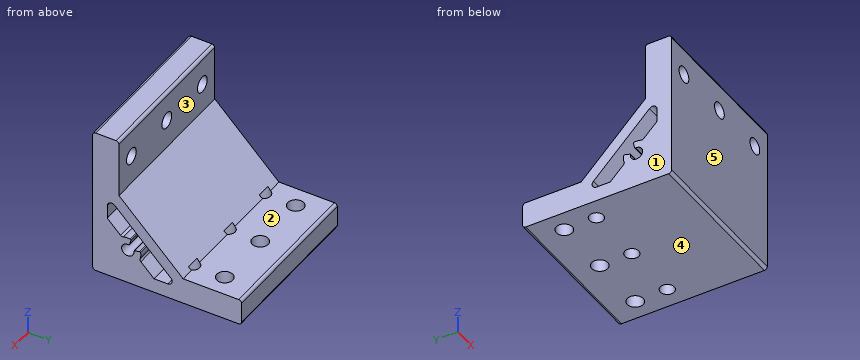
from build123d import *

# Parameters (mm, degrees)
BOSS_EXTRUDE1_DEPTH      = 27
BOSS_EXTRUDE1_DEPTH_BACK = 27
SKETCH6_R                = 2.75
CUT_EXTRUDE5_DEPTH       = 10
SKETCH7_R                = 2.75
CUT_EXTRUDE6_DEPTH       = 10
SKETCH9_R                = 2.4
CUT_EXTRUDE7_DEPTH       = 10


with BuildPart() as part:
    # Sketch1 → Boss-Extrude1 (new body, two sides)
    with BuildSketch(Plane(origin=(0, 0, 0), x_dir=(0, 0, -1), z_dir=(1, 0, 0))) as boss_extrude1_sk:
        with BuildLine():
            Line((-50, 0), (-1, 0))
            ThreePointArc((-1, 0), (-0.292893219, 0.292893219), (0, 1))
            Line((0, 1), (0, 50))
            ThreePointArc((0, 50), (-0.292893219, 50.707106781), (-1, 51))
            Line((-1, 51), (-8, 51))
            ThreePointArc((-8, 51), (-8.707106781, 50.707106781), (-9, 50))
            Line((-9, 50), (-9, 31))
            Line((-9, 31), (-31, 9))
            Line((-31, 9), (-50, 9))
            ThreePointArc((-50, 9), (-50.707106781, 8.707106781), (-51, 8))
            Line((-51, 8), (-51, 1))
            ThreePointArc((-51, 1), (-50.707106781, 0.292893219), (-50, 0))
        make_face()
        with BuildLine():
            Line((-25.721825407, 5), (-20.999285733, 5))
            Line((-20.999285733, 5), (-16.494036438, 9.505249294))
            ThreePointArc((-16.494036438, 9.505249294), (-16.226979866, 9.987090789), (-16.255625497, 10.537245192))
            ThreePointArc((-16.255625497, 10.537245192), (-16.488859314, 11.683547702), (-16.418755424, 12.851234691))
            ThreePointArc((-16.418755424, 12.851234691), (-16.283360667, 13.048766752), (-16.046526031, 13.084263382))
            Line((-16.046526031, 13.084263382), (-14.300039569, 12.616293745))
            ThreePointArc((-14.300039569, 12.616293745), (-14.127781033, 12.492491496), (-14.080474622, 12.285701498))
            ThreePointArc((-14.080474622, 12.285701498), (-10.515075745, 10.515075774), (-12.285701539, 14.080474617))
            ThreePointArc((-12.285701539, 14.080474617), (-12.492491514, 14.127781045), (-12.616293745, 14.300039569))
            Line((-12.616293745, 14.300039569), (-13.084263382, 16.046526031))
            ThreePointArc((-13.084263382, 16.046526031), (-13.048766728, 16.283360705), (-12.851234602, 16.418755442))
            ThreePointArc((-12.851234602, 16.418755442), (-11.683774102, 16.488875269), (-10.537674556, 16.255773055))
            ThreePointArc((-10.537674556, 16.255773055), (-9.987311976, 16.226928716), (-9.505249294, 16.494036438))
            Line((-9.505249294, 16.494036438), (-5, 20.999285733))
            Line((-5, 20.999285733), (-5, 25.721825407))
            ThreePointArc((-5, 25.721825407), (-5.925974851, 27.107644706), (-7.560660172, 26.782485579))
            Line((-7.560660172, 26.782485579), (-26.782485579, 7.560660172))
            ThreePointArc((-26.782485579, 7.560660172), (-27.107644706, 5.925974851), (-25.721825407, 5))
        make_face(mode=Mode.SUBTRACT)
    extrude(amount=BOSS_EXTRUDE1_DEPTH)
    extrude(boss_extrude1_sk.sketch, amount=-BOSS_EXTRUDE1_DEPTH_BACK)

    # Sketch6 → Cut-Extrude5 (cut, through all)
    with BuildSketch(Plane.XY.offset(9)):
        with Locations((-20, 41)):
            Circle(SKETCH6_R)
        with Locations((0, 41)):
            Circle(SKETCH6_R)
        with Locations((20, 41)):
            Circle(SKETCH6_R)
    extrude(amount=-CUT_EXTRUDE5_DEPTH, mode=Mode.SUBTRACT)

    # Sketch7 → Cut-Extrude6 (cut, through all)
    with BuildSketch(Plane(origin=(0, 9, 0), x_dir=(-1, 0, 0), z_dir=(0, 1, 0))):
        with Locations((20, 41)):
            Circle(SKETCH7_R)
        with Locations((0, 41)):
            Circle(SKETCH7_R)
        with Locations((-20, 41)):
            Circle(SKETCH7_R)
    extrude(amount=-CUT_EXTRUDE6_DEPTH, mode=Mode.SUBTRACT)

    # Sketch9 → Cut-Extrude7 (cut)
    with BuildSketch(Plane(origin=(0, 0, 0), x_dir=(-1, 0, 0), z_dir=(0, 0, -1))):
        with Locations((20, 30)):
            Circle(SKETCH9_R)
        with Locations((-20, 30)):
            Circle(SKETCH9_R)
        with Locations((0, 30)):
            Circle(SKETCH9_R)
    extrude(amount=-CUT_EXTRUDE7_DEPTH, mode=Mode.SUBTRACT)


solid = part.part
The listing builds one solid part. Answer for the finished solid, in the listing's coordinates (mm). Face numbers are marked on the shaded views. A direction names the side the tool comes from. Coordinates: 2 decimals unless noted, no trailing zeros. Write each loop counter-clockwise with the first axis right and the second up, starting at its lowest first coordinate (ties: lowest second). Pieces come first, ordered by that corner, then holes. Notation, with made-up numbers: M 49.25,55 L 103.25,55 A11 ccw 103.25,76 Z; hole C 85.25,88 d3. An arc over 180 degrees is marked long. Use one line per item in the form item = value.
Item 1: Find section A-A, the plane z = 41. Give the vertices of the cut face in (x, y).
Model answer:
outline = M -27,0 L -22.75,0 L -22.75,9 L -27,9 Z; M -17.25,0 L -2.75,0 L -2.75,9 L -17.25,9 Z; M 2.75,0 L 17.25,0 L 17.25,9 L 2.75,9 Z; M 22.75,0 L 27,0 L 27,9 L 22.75,9 Z
Item 2: Find the intervals of material crossed by probe 1 along Y at (x, z) = (20, 2); probe 2 along Z at (x, y) = (-18, 6.5); probe 3 along Y at (x, z) = (1.5, 8.5), in increasing order.
Model answer:
probe_1 = 0 to 27.6, 32.4 to 38.25, 43.75 to 51
probe_2 = 0 to 19.5, 27.22 to 39.11, 42.89 to 51
probe_3 = 0 to 17.5, 25.84 to 28.13, 31.87 to 38.7, 43.3 to 50.87
Item 3: Find section D-D, the plane z = 32. Give the vertices of the cut face in (x, y), plus the area to 3 significant figures.
Model answer:
outline = M -27,0 L 27,0 L 27,9 L -27,9 Z
area = 486 mm2
Item 4: The mould has two halves that part along Y. Classify the marked faces 3, 4 and 5: released by +Y, released by -Y, zero draft, split by the parting line, or undercut.
Model answer:
face_3 = released by +Y
face_4 = zero draft
face_5 = released by -Y
Item 5: For the marked faces 1 and 2, determine the directions among +Z, -Z, +X, -X, +Y, -Y from which every point of the face is accessible in a straight line to the end or side of a thin tool.
Model answer:
face_1 = +Z, -Z, -X, +Y, -Y
face_2 = +Z, +X, -X, +Y
Item 6: Given P1, Ø6.5, axis at y = 12, z = 12, coming from the +X side; P2, Ø2.5, axis at x = -7.5, y = 22.5, coming from the +Z side; P3, Ø0.7, axis at x = -20, y = 29, coming from the -Z side; P4, Ø15, axis at x = -2.5, y = 43.5, coming from the +Z side, each flat-ended and moving along its own axis, determine where each tip first touches the part or whether it passes through.
Model answer:
P1 = 27
P2 = 18.75
P3 = 10
P4 = 9
